Input: part model. Units: mm. Frame: model coordinates. Give positions to 0.01 mm unless a question says otherwise; leave off trailing zeros. Write each loop counter-clockwise with the first axis right and the second up, starting at its lowest first coordinate (ties: lowest second). Pieces come first, ordered by that corner, then holes. Notation, with made-up numbers: M 54.25,50.25 L 63.25,50.25 A21 ccw 63.25,60.25 Z; hole C 29,-39.5 d3. An arc over 180 degrees is marked long. Use CSV: the item, a comma, the result in double quotes. Start each with the question number.
from build123d import *

# Parameters (mm, degrees)
SKETCH1_W                 = 186
SKETCH1_H                 = 123
SKETCH1_R                 = 27.35
BOSS_EXTRUDE1_DEPTH       = 3
FILLET1_R                 = 10
TAP_DRILL_FOR_4_40_TAP1_D = 2.2606


with BuildPart() as part:
    # Sketch1 → Boss-Extrude1 (new body)
    with BuildSketch(Plane(origin=(0, 0, 0), x_dir=(1, 0, 0), z_dir=(0, 1, 0))):
        Rectangle(SKETCH1_W, SKETCH1_H)
        with Locations(Location((-63, 31.5, 0), (0, 0, 270))):
            Circle(SKETCH1_R, mode=Mode.SUBTRACT)
        with Locations(Location((0, 31.5, 0), (0, 0, 270))):
            Circle(SKETCH1_R, mode=Mode.SUBTRACT)
        with Locations(Location((63, 31.5, 0), (0, 0, 270))):
            Circle(SKETCH1_R, mode=Mode.SUBTRACT)
        with Locations(Location((0, -31.5, 0), (0, 0, 270))):
            Circle(SKETCH1_R, mode=Mode.SUBTRACT)
        with Locations(Location((63, -31.5, 0), (0, 0, 270))):
            Circle(SKETCH1_R, mode=Mode.SUBTRACT)
        with Locations(Location((-63, -31.5, 0), (0, 0, 270))):
            Circle(SKETCH1_R, mode=Mode.SUBTRACT)
    extrude(amount=BOSS_EXTRUDE1_DEPTH)

    # Fillet1
    fillet1_edges = [part.edges().sort_by_distance(p)[0] for p in [
        (-93, 1.5, -61.5),
        (93, 1.5, -61.5),
        (93, 1.5, 61.5),
        (-93, 1.5, 61.5),
    ]]
    fillet(fillet1_edges, radius=FILLET1_R)

    # Tap Drill for #4-40 Tap1 (through all)
    with Locations(Plane(origin=(0, 3, 0), x_dir=(1, 0, 0), z_dir=(0, 1, 0))):
        with Locations((0, 0), (31.5, 51.5), (-31.5, 51.5), (-31.5, -51.5), (31.5, -51.5)):
            Hole(TAP_DRILL_FOR_4_40_TAP1_D / 2)


solid = part.part
Q1. Section B-B, the plane z = -31.5. Return the cut outline in (x, y).
Q2. Material intervals for L1, parallel to X at y = 2.75, z = -33; L2, parallel to Z at x = -31.5, y = 1.3; L3, parallel to X at y = 1.7, z = -19.5, sorted ascending. Write a range as [from, to].
Q3. Section A-A, the plane x = -63. Return the cut outline in (y, z).
Q4. Section D-D, the plane x = 67.5. Return the cut outline in (y, z), and give its area (3 significant figures).
Q5. First-contact query: pin 1 Ø2.5 at (x, z) = (-31.5, 51.5) entering from +Y. Flat tip, straight axial feed; report the tip coordinate or a pass-through.
Q6. Section C-C, the plane z = 26. Return the cut outline in (x, y).
Q7. Pull-direction query (X, two-part tool) for faces 1 (the cylindrical face through (-87.264, 1.479, -18.88)), 2 (the flat face through (-7, 0, 0)), 3 (the cylindrical face through (89.99, 1.52, 58.65)), 4 (the cylindrical face through (8.215, 1.479, -5.413)); classes: released by +X, released by -X, zero draft, split by the parting line, or undercut.
Check result:
1,outline,"M -93,0 L -90.35,0 L -90.35,3 L -93,3 Z; M -35.65,0 L -27.35,0 L -27.35,3 L -35.65,3 Z; M 27.35,0 L 35.65,0 L 35.65,3 L 27.35,3 Z; M 90.35,0 L 93,0 L 93,3 L 90.35,3 Z"
2,L1,"x = [-93, -90.31], [-35.69, -27.31], [27.31, 35.69], [90.31, 93]"
2,L2,"z = [-61.5, -52.63], [-50.37, 50.37], [52.63, 61.5]"
2,L3,"x = [-93, -87.58], [-38.42, -24.58], [24.58, 38.42], [87.58, 93]"
3,outline,"M 0,-61.5 L 3,-61.5 L 3,-58.85 L 0,-58.85 Z; M 0,-4.15 L 3,-4.15 L 3,4.15 L 0,4.15 Z; M 0,58.85 L 3,58.85 L 3,61.5 L 0,61.5 Z"
4,outline,"M 0,-61.5 L 3,-61.5 L 3,-58.48 L 0,-58.48 Z; M 0,-4.52 L 3,-4.52 L 3,4.52 L 0,4.52 Z; M 0,58.48 L 3,58.48 L 3,61.5 L 0,61.5 Z"
4,area,"45.3 mm²"
5,pin 1,"stops at y = 3"
6,outline,"M -93,0 L -89.79,0 L -89.79,3 L -93,3 Z; M -36.21,0 L -26.79,0 L -26.79,3 L -36.21,3 Z; M 26.79,0 L 36.21,0 L 36.21,3 L 26.79,3 Z; M 89.79,0 L 93,0 L 93,3 L 89.79,3 Z"
7,face 1,"undercut"
7,face 2,"zero draft"
7,face 3,"released by +X"
7,face 4,"undercut"
